from build123d import *

# Parameters (mm, degrees)
CROQUIS1_W              = 24
CROQUIS1_H              = 4
SALIENTE_EXTRUIR1_DEPTH = 3
CROQUIS4_R              = 1.15
CORTAR_EXTRUIR2_DEPTH   = 25.515301344
CROQUIS3_R              = 1.05
SALIENTE_EXTRUIR3_DEPTH = 2


with BuildPart() as part:
    # Croquis1 → Saliente-Extruir1 (new body)
    with BuildSketch(Plane.XY):
        with Locations((12, -2)):
            Rectangle(CROQUIS1_W, CROQUIS1_H)
    extrude(amount=SALIENTE_EXTRUIR1_DEPTH)

    # Croquis4 → Cortar-Extruir2 (cut, through all)
    with BuildSketch(Plane.XY.offset(3)):
        with Locations((2.75, -2)):
            Circle(CROQUIS4_R)
    extrude(amount=-CORTAR_EXTRUIR2_DEPTH, mode=Mode.SUBTRACT)

    # Croquis3 → Saliente-Extruir3 (add)
    with BuildSketch(Plane(origin=(0, 0, 0), x_dir=(-1, 0, 0), z_dir=(0, 0, -1))):
        with Locations(Location((-20, -2, 0), (0, 0, 180))):
            Circle(CROQUIS3_R)
    extrude(amount=SALIENTE_EXTRUIR3_DEPTH)


solid = part.part
Geometry: final body of the model. Coordinates: model frame, mm. A direction names the side the tool comes from. Give positions to 0.01 mm unless a question says otherwise; leave off trailing zeros. Write each loop counter-clockwise with the first axis right and the second up, starting at its lowest first coordinate (ties: lowest second). Pieces come first, ordered by that corner, then holes. Notation, with made-up numbers: (86, 40.5) -> (116, 40.5) arc R11 cw to (116, 46.5) -> close; hole circle Ø1 at (46, -21.75). An arc over 180 degrees is marked (long way). Answer as a JSON object with one key per item and string values.
1. Cut plane B-B on y = -2. Output: boundary loops of the cut face in (x, z).
Ans:
{"outline": "(0, 0) -> (1.6, 0) -> (1.6, 3) -> (0, 3) -> close; (3.9, 0) -> (18.95, 0) -> (18.95, -2) -> (21.05, -2) -> (21.05, 0) -> (24, 0) -> (24, 3) -> (3.9, 3) -> close"}
2. Ray query, probe 1 along Y at (x, z) = (2.75, 1.9); probe 2 along Z at (x, y) = (4.25, -0.85); probe 3 along X at (y, z) = (-1.55, 1.1). Return the intervals inside material, ascending. Write a range as from..to.
Ans:
{"probe 1": "y = -4..-3.15, -0.85..0", "probe 2": "z = 0..3", "probe 3": "x = 0..1.69, 3.81..24"}
3. Mould query, pull axis Y, two halves, no side actions, for faces 1 (the flat face through (24, -2, 1)), 2 (the flat face through (12, -4, 1)), 3 (the cylindrical face through (1.84, -2.7, 1.52)). Classes: pulls with the +Y half, pulls with the -Y half, needs draft (parallel to the pull), parting line crosses it, or undercut.
Ans:
{"face 1": "needs draft", "face 2": "pulls with the -Y half", "face 3": "undercut"}
4. Cut plane A-A on x = 2.75. Output: boundary loops of the cut face in (y, z), and give its area (3 significant figures).
Ans:
{"outline": "(-4, 0) -> (-3.15, 0) -> (-3.15, 3) -> (-4, 3) -> close; (-0.85, 0) -> (0, 0) -> (0, 3) -> (-0.85, 3) -> close", "area": "5.10 mm^2"}
5. Contact query for flat-ended pins moving along their axis: pin 1 (2 mm diameter, centred on x = 15, y = -0.5, fed in from -Z); pin 2 (1.8 mm diameter, centred on x = 2.75, y = -2, fed in from +Z). Output: stop coordinate, or through.
Ans:
{"pin 1": "stops at z = 0", "pin 2": "passes through"}
6. Cut plane D-D on x = 20. Output: boundary loops of the cut face in (y, z).
Ans:
{"outline": "(-4, 0) -> (-3.05, 0) -> (-3.05, -2) -> (-0.95, -2) -> (-0.95, 0) -> (0, 0) -> (0, 3) -> (-4, 3) -> close"}
7. Access query for faces 4 (the cylindrical face through (18.95, -2.05, -0.99)), 5 (the flat face through (20, -2, -2)). Directions: +Z, -Z, +X, -X, +Y, -Y. A direction counts if a zero-diameter tool reaches every point of the face in a straight line with its end or side. Return the directions, or none.
Ans:
{"face 4": "-Z", "face 5": "-Z, +X, -X, +Y, -Y"}
8. Cut plane C-C on z = 1.45. Output: boundary loops of the cut face in (x, y), and give its area (3 significant figures).
Ans:
{"outline": "(0, -4) -> (24, -4) -> (24, 0) -> (0, 0) -> close; hole circle Ø2.3 at (2.75, -2)", "area": "91.8 mm^2"}
